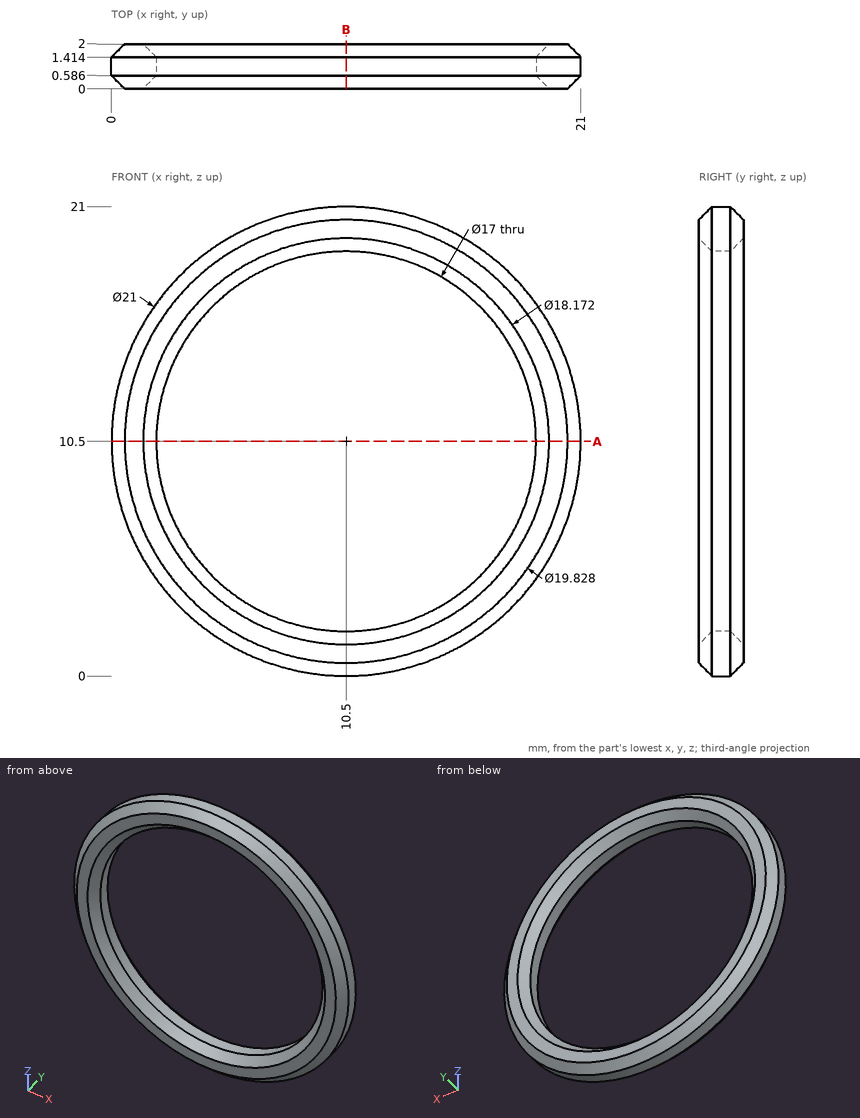
Verification items for this drawing (mm, ordinates from the low corner). Round coordinates to 2 decimals unless told otherwise and drop trailing zeros. Order: outer loops, then holes, each group sorted by start corner. A loop starts at its lowest first (then second) coordinate and runs counter-clockwise, first axis right, second up. Notation, with made-up numbers: M 28,30.25 L 56,30.25 A21 ccw 56,50.25 Z; hole C 46.25,66.5 d8. An arc over 180 degrees is marked long. Answer in a Markdown table with one row per item. Add a question column.
Item 1: Sectioned sample at A-A, the plane z = 10.5. Enter the section's corners in (x, y) (1 decimal).
Item 2: Sectioned sample at B-B, the plane x = 10.5. Enter the section's corners in (y, z) (1 decimal).
Item 3: Depth check by flat-ended pin: pin 1 Ø1.5 at (x, z) = (11.5, 4) entering from +Y. Enter the tip coordinate at first touch or a pass-through.
Item 4: Material ranges on L1, parallel to X at y = 1, z = 10.5; L2, parallel to X at y = 0.75, z = 16.5 (1 decimal), recorded low to high. Write a range as [from, to].
Filled in:
| question | item | result |
|---|---|---|
| 1 | outline | M 0,0.6 L 0.6,0 L 1.4,0 L 2,0.6 L 2,1.4 L 1.4,2 L 0.6,2 L 0,1.4 Z; M 19,0.6 L 19.6,0 L 20.4,0 L 21,0.6 L 21,1.4 L 20.4,2 L 19.6,2 L 19,1.4 Z |
| 2 | outline | M 0,0.6 L 0.6,0 L 1.4,0 L 2,0.6 L 2,1.4 L 1.4,2 L 0.6,2 L 0,1.4 Z; M 0,19.6 L 0.6,19 L 1.4,19 L 2,19.6 L 2,20.4 L 1.4,21 L 0.6,21 L 0,20.4 Z |
| 3 | pin 1 | passes through |
| 4 | L1 | x = [0, 2], [19, 21] |
| 4 | L2 | x = [1.9, 4.5], [16.5, 19.1] |
